Source: CAD feature listing. Evaluate the final solid. Frame: model axes, mm. A direction names the side the tool comes from. Coordinates: 2 decimals unless noted, no trailing zeros. Write each loop counter-clockwise with the first axis right and the second up, starting at its lowest first coordinate (ties: lowest second). Pieces come first, ordered by that corner, then holes. Notation, with made-up numbers: (-26.5, -27.5) -> (3.5, -27.5) arc R16 ccw to (3.5, -0.5) -> close; hole circle Ø8 at (-2, 85). An arc over 180 degrees is marked (long way). One line per item, written item: value. Start each with the question number.
1. Section query D-D, the plane z = 3.75. State how many separate pieces and enclosed holes the cut face has, and give its area (3 significant figures).
2. Access query for faces 1 (the flat face through (-6.985, 32, 3)), 2 (the cylindrical face through (29.403, -1.698, 3.444)). Directions: +Z, -Z, +X, -X, +Y, -Y. A direction counts if a zero-diameter tool reaches every point of the face in a straight line with its end or side. Return the directions, or none.
3. Section query C-C, the plane y = 18.5. Output: boundary loops of the cut face in (x, z) (3 decimals), and give its area (3 significant figures).
4. Section query A-A, the plane x = 0. Output: boundary loops of the cut face in (y, z) (1 decimal), and give its area (3 significant figures).
5. Section query B-B, the plane y = 6. Output: boundary loops of the cut face in (x, z) (3 decimals), and give its area (3 significant figures).
6. Line query: line 1 (X direction, y = 35, z = 6.75) (3 decimals); line 2 (Y direction, x = 32.5, z = 1.25); line 3 (X direction, y = 51, z = 1) (3 decimals). Output: solid intervals per line, ascending.
7. First-contact query: P1, Ø8.5, axis at x = 41.656, y = 0, coming from the +Z side (3 decimals). Flat tip, straight axial feed; report the tip coordinate or a pass-through.
8. Mould query, pull axis Y, two halves, no side actions, for faces 3 (the flat face through (18.288, 55, 3)), 4 (the cylindrical face through (-6.03, -6.78, 3.44)), 5 (the cylindrical face through (47.7, 69.5, 3.4)), 6 (the flat face through (31.623, 31, 3)). Classes: released by +Y, released by -Y, zero draft, split by the parting line, or undercut.
Autodesk Inventor part; units mm, degrees
ref_plane "YZ Plane" through (0, 0, 0) normal (1, 0, 0) x (0, 1, 0)
ref_plane "XZ Plane" through (0, 0, 0) normal (0, 1, 0) x (-1, 0, 0)
ref_plane "XY Plane" through (0, 0, 0) normal (0, 0, 1) x (1, 0, 0)
sketch "Sketch1" plane through (0, 0, 0) normal (0, 0, 1) x (1, 0, 0)
  line L0 (-3.81, -7.6835) -> (45.466, -7.6835)
  line L1 (48.641, -4.5085) -> (48.641, 67.2465)
  line L2 (45.466, 70.4215) -> (-3.81, 70.4215)
  line L3 (-6.985, 67.2465) -> (-6.985, -4.5085)
  arc A0 (45.466, -7.6835) -> (48.641, -4.5085) centre (45.466, -4.5085) ccw
  arc A1 (-6.985, -4.5085) -> (-3.81, -7.6835) centre (-3.81, -4.5085) ccw
  line L4 (31.623, 19.304) -> (31.623, 43.434)
  line L5 (10.033, 43.434) -> (10.033, 19.304)
  line L6 (18.288, -7.6835) -> (23.368, -7.6835)
  line L7 (23.368, 70.4215) -> (18.288, 70.4215)
  arc A2 (-1.905, 55.0979) -> (7.874, 62.738) centre (0, 62.738) ccw
  arc A3 (33.782, 62.738) -> (43.561, 55.0979) centre (41.656, 62.738) ccw
  arc A4 (43.561, 7.6401) -> (34.2249, -2.6035) centre (41.656, 0) ccw
  arc A5 (7.4311, -2.6035) -> (-1.905, 7.6401) centre (0, 0) ccw
  line L8 (34.2249, -2.6035) -> (31.623, -2.6035)
  line L9 (10.033, -2.6035) -> (7.4311, -2.6035)
  line L10 (31.623, 43.434) -> (26.543, 43.434)
  line L11 (15.113, 43.434) -> (10.033, 43.434)
  line L12 (10.033, 19.304) -> (15.113, 19.304)
  line L13 (26.543, 19.304) -> (31.623, 19.304)
  line L14 (23.368, 46.609) -> (23.368, 62.738)
  line L15 (18.288, 62.738) -> (18.288, 46.609)
  line L16 (23.368, -2.6035) -> (23.368, 16.129)
  line L17 (18.288, 16.129) -> (18.288, -2.6035)
  line L18 (18.288, -2.6035) -> (23.368, -2.6035)
  line L19 (28.448, 51.689) -> (28.448, 59.563)
  line L20 (40.386, 48.514) -> (31.623, 48.514)
  line L21 (13.208, 59.563) -> (13.208, 51.689)
  line L22 (10.033, 48.514) -> (1.27, 48.514)
  line L23 (13.208, 11.049) -> (13.208, 0.5715)
  line L24 (1.27, 14.224) -> (10.033, 14.224)
  line L25 (31.623, 14.224) -> (40.386, 14.224)
  line L26 (28.448, 0.5715) -> (28.448, 11.049)
  line L27 (-1.905, 7.6401) -> (-1.905, 11.049)
  line L28 (-1.905, 51.689) -> (-1.905, 55.0979)
  line L29 (43.561, 55.0979) -> (43.561, 51.689)
  line L30 (43.561, 11.049) -> (43.561, 7.6401)
  line L31 (43.561, 22.479) -> (43.561, 40.259)
  line L32 (-1.905, 40.259) -> (-1.905, 22.479)
  line L33 (4.953, 40.259) -> (4.953, 22.479)
  line L34 (36.703, 22.479) -> (36.703, 40.259)
  line L35 (1.27, 43.434) -> (1.778, 43.434)
  line L36 (1.778, 19.304) -> (1.27, 19.304)
  line L37 (39.878, 43.434) -> (40.386, 43.434)
  line L38 (40.386, 19.304) -> (39.878, 19.304)
  arc A6 (10.033, 48.514) -> (13.208, 51.689) centre (10.033, 51.689) ccw
  arc A7 (28.448, 51.689) -> (31.623, 48.514) centre (31.623, 51.689) ccw
  arc A8 (31.623, 14.224) -> (28.448, 11.049) centre (31.623, 11.049) ccw
  arc A9 (13.208, 11.049) -> (10.033, 14.224) centre (10.033, 11.049) ccw
  arc A10 (1.27, 14.224) -> (-1.905, 11.049) centre (1.27, 11.049) ccw
  arc A11 (10.033, -2.6035) -> (13.208, 0.5715) centre (10.033, 0.5715) ccw
  arc A12 (28.448, 0.5715) -> (31.623, -2.6035) centre (31.623, 0.5715) ccw
  arc A13 (43.561, 11.049) -> (40.386, 14.224) centre (40.386, 11.049) ccw
  arc A14 (40.386, 48.514) -> (43.561, 51.689) centre (40.386, 51.689) ccw
  arc A15 (-1.905, 51.689) -> (1.27, 48.514) centre (1.27, 51.689) ccw
  arc A16 (23.368, 46.609) -> (26.543, 43.434) centre (26.543, 46.609) ccw
  arc A17 (15.113, 43.434) -> (18.288, 46.609) centre (15.113, 46.609) ccw
  arc A18 (18.288, 16.129) -> (15.113, 19.304) centre (15.113, 16.129) ccw
  arc A19 (26.543, 19.304) -> (23.368, 16.129) centre (26.543, 16.129) ccw
  arc A20 (36.703, 22.479) -> (39.878, 19.304) centre (39.878, 22.479) ccw
  arc A21 (40.386, 19.304) -> (43.561, 22.479) centre (40.386, 22.479) ccw
  arc A22 (43.561, 40.259) -> (40.386, 43.434) centre (40.386, 40.259) ccw
  arc A23 (39.878, 43.434) -> (36.703, 40.259) centre (39.878, 40.259) ccw
  arc A24 (1.27, 43.434) -> (-1.905, 40.259) centre (1.27, 40.259) ccw
  arc A25 (4.953, 40.259) -> (1.778, 43.434) centre (1.778, 40.259) ccw
  arc A26 (1.778, 19.304) -> (4.953, 22.479) centre (1.778, 22.479) ccw
  arc A27 (-1.905, 22.479) -> (1.27, 19.304) centre (1.27, 22.479) ccw
  line L39 (7.874, 62.738) -> (10.033, 62.738)
  line L40 (18.288, 62.738) -> (23.368, 62.738)
  line L41 (31.623, 62.738) -> (33.782, 62.738)
  arc A28 (13.208, 59.563) -> (10.033, 62.738) centre (10.033, 59.563) ccw
  arc A29 (31.623, 62.738) -> (28.448, 59.563) centre (31.623, 59.563) ccw
  circle A30 centre (0, 62.738) radius 3.302
  circle A31 centre (41.656, 62.738) radius 3.302
  circle A32 centre (0, 0) radius 3.302
  circle A33 centre (41.656, 0) radius 3.302
  arc A34 (-3.81, 70.4215) -> (-6.985, 67.2465) centre (-3.81, 67.2465) ccw
  arc A35 (48.641, 67.2465) -> (45.466, 70.4215) centre (45.466, 67.2465) ccw
  point P0 (20.828, 31.369)
  point P1 (-6.985, 70.4215)
  point P2 (48.641, 70.4215)
  point P3 (23.368, 43.434)
  point P4 (18.288, 43.434)
  point P5 (18.288, 19.304)
  point P6 (23.368, 19.304)
  point P7 (-1.905, 14.224)
  point P8 (43.561, 48.514)
  point P9 (43.561, 14.224)
  point P10 (-1.905, 48.514)
  point P11 (13.208, 65.3415)
  point P12 (28.448, 65.3415)
  point P13 (13.208, -2.6035)
  point P14 (28.448, -2.6035)
  point P15 (28.448, 48.514)
  point P16 (13.208, 48.514)
  point P17 (13.208, 14.224)
  point P18 (28.448, 14.224)
  point P19 (-1.905, 19.304)
  point P20 (43.561, 43.434)
  point P21 (43.561, 19.304)
  point P22 (-1.905, 43.434)
  point P23 (4.953, 43.434)
  point P24 (4.953, 19.304)
  point P25 (36.703, 19.304)
  point P26 (36.703, 43.434)
  point P27 (28.448, 62.738)
  point P28 (13.208, 62.738)
  dimension "d32" = 3.175
  dimension "d37" = 6.604
  dimension "d38" = 6.604
  dimension "d39" = 6.604
  dimension "d40" = 6.604
  dimension "d76" = 3.175
extrude "Extrusion1" add sketch "Sketch1" along normal blind 6.985
properties part number "LED Riser"
Computed values:
1. separate pieces: 1
1. enclosed holes: 11
1. area: 2,540 mm²
2. face 1: +Z, -Z, -X, +Y, -Y
2. face 2: +Z, -Z
3. outline: (-6.985, 0) -> (17.225, 0) -> (17.225, 6.985) -> (-6.985, 6.985) -> close; (24.431, 0) -> (48.641, 0) -> (48.641, 6.985) -> (24.431, 6.985) -> close
3. area: 338 mm²
4. outline: (-7.7, 0) -> (-3.3, 0) -> (-3.3, 7) -> (-7.7, 7) -> close; (3.3, 0) -> (7.9, 0) -> (7.9, 7) -> (3.3, 7) -> close; (14, 0) -> (19.6, 0) -> (19.6, 7) -> (14, 7) -> close; (43.2, 0) -> (48.8, 0) -> (48.8, 7) -> (43.2, 7) -> close; (54.9, 0) -> (59.4, 0) -> (59.4, 7) -> (54.9, 7) -> close; (66, 0) -> (70.4, 0) -> (70.4, 7) -> (66, 7) -> close
4. area: 203 mm²
5. outline: (-6.985, 0) -> (5.099, 0) -> (5.099, 6.985) -> (-6.985, 6.985) -> close; (13.208, 0) -> (18.288, 0) -> (18.288, 6.985) -> (13.208, 6.985) -> close; (23.368, 0) -> (28.448, 0) -> (28.448, 6.985) -> (23.368, 6.985) -> close; (36.557, 0) -> (48.641, 0) -> (48.641, 6.985) -> (36.557, 6.985) -> close
5. area: 240 mm²
6. line 1: x = -6.985 to -1.905, 4.953 to 10.033, 31.623 to 36.703, 43.561 to 48.641
6. line 2: y = -7.68 to -2.6, 14.22 to 48.51, 62.74 to 70.42
6. line 3: x = -6.985 to -1.829, 13.132 to 18.288, 23.368 to 28.524, 43.485 to 48.641
7. P1: stops at z = 6.985
8. face 3: undercut
8. face 4: released by -Y
8. face 5: released by +Y
8. face 6: undercut
